Read the model definition and answer for the solid it produces. Units are mm, in the model's axes. Face numbers are marked on the shaded views. Coordinates: 2 decimals unless noted, no trailing zeros. Write each loop counter-clockwise with the first axis right and the second up, starting at its lowest first coordinate (ties: lowest second). Pieces come first, ordered by that corner, then holes. Notation, with made-up numbers: M 55.25,84.25 L 101.25,84.25 A19 cw 101.25,109.25 Z; hole C -15,6.5 d8. An arc over 180 degrees is marked long. Use a Markdown table: item, result. Add a question column.
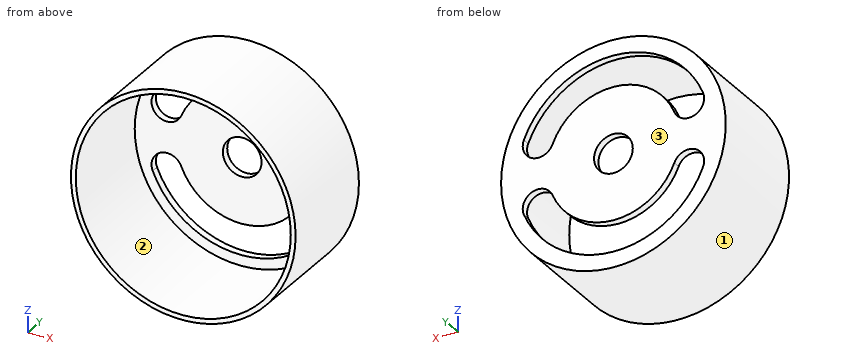
from build123d import *

# Parameters (mm, degrees)
F0_R     = 29
F1_DEPTH = 29
F2_R     = 27.75
F3_DEPTH = 27
F5_DEPTH = 2
F6_R     = 5
F7_DEPTH = 2


with BuildPart() as f1:
    # F0 (on Front) → F1 (new body)
    with BuildSketch(Plane.XZ):
        Circle(F0_R)
    extrude(amount=F1_DEPTH)

    # F2 (on face) → F3 (cut)
    with BuildSketch(Plane.XZ.offset(29)):
        Circle(F2_R)
    extrude(amount=-F3_DEPTH, mode=Mode.SUBTRACT)

    # F4 (on face) → F5 (cut)
    with BuildSketch(Plane(origin=(0, 0, 0), x_dir=(-1, 0, 0), z_dir=(0, 1, 0))):
        with BuildLine():
            ThreePointArc((-15.718109, -6.47619), (-20.940297, -4.301621), (-23.114866, -9.52381))
            ThreePointArc((-23.114866, -9.52381), (0, -25), (23.114866, -9.52381))
            ThreePointArc((23.114866, -9.52381), (20.940297, -4.301621), (15.718109, -6.47619))
            ThreePointArc((15.718109, -6.47619), (0, -17), (-15.718109, -6.47619))
        make_face()
        with BuildLine():
            ThreePointArc((23.114866, 9.52381), (0, 25), (-23.114866, 9.52381))
            ThreePointArc((-23.114866, 9.52381), (-20.940297, 4.301621), (-15.718109, 6.47619))
            ThreePointArc((-15.718109, 6.47619), (0, 17), (15.718109, 6.47619))
            ThreePointArc((15.718109, 6.47619), (20.940297, 4.301621), (23.114866, 9.52381))
        make_face()
    extrude(amount=-F5_DEPTH, mode=Mode.SUBTRACT)

    # F6 (on face) → F7 (cut)
    with BuildSketch(Plane(origin=(0, 0, 0), x_dir=(-1, 0, 0), z_dir=(0, 1, 0))):
        Circle(F6_R)
    extrude(amount=-F7_DEPTH, mode=Mode.SUBTRACT)


solid = f1.part
Item 1: Consider probe 1 along Z at (x, y) = (0, -0.8); probe 2 along Z at (x, y) = (0, -20.75); probe 3 along Z at (x, y) = (-24.5, -21.5). Determine where each line is inside the solid, lowest interval first.
Item 2: Find section D-D on x = -8. Give the vertices of the cut face in (y, z), then the cut area to 3 significant figures.
Item 3: Find section C-C on z = 8. Give the vertices of the cut face in (x, y).
Item 4: Determine the mould class of the marked faces 1, 2 and 3 for opening direction X: pulls with the +X half, pulls with the -X half, needs draft (parallel to the pull), parting line crosses it, or undercut.
Item 5: Find section A-A on z = 0. Give the vertices of the cut face in (x, y), then the cut area to 4 significant figures.
Item 6: Each of these flat-tipped pins is pushed along its axis until it touches: pin 1 (5 mm diameter, centred on x = -19, y = -22, fed in from +Z); pin 2 (12 mm diameter, centred on y = -12.5, z = 15, fed in from +X); pin 3 (4 mm diameter, centred on y = -22, z = -12.5, fed in from +X). Where does it stop, or does it pass through?
Item 7: Find section B-B on x = 0. Give the vertices of the cut face in (y, z), then the cut area to 4 significant figures.
Geometry says:
| question | item | result |
|---|---|---|
| 1 | probe 1 | z = -29 to -25, -17 to -5, 5 to 17, 25 to 29 |
| 1 | probe 2 | z = -29 to -27.75, 27.75 to 29 |
| 1 | probe 3 | z = -15.52 to -13.03, 13.03 to 15.52 |
| 2 | outline | M -29,-27.87 L 0,-27.87 L 0,-23.69 L -2,-23.69 L -2,-26.57 L -29,-26.57 Z; M -29,26.57 L -2,26.57 L -2,23.69 L 0,23.69 L 0,27.87 L -29,27.87 Z; M -2,-15 L 0,-15 L 0,15 L -2,15 Z |
| 2 | area | 147 mm2 |
| 3 | outline | M -27.87,-29 L -26.57,-29 L -26.57,-2 L -23.42,-2 L -23.42,0 L -27.87,0 Z; M -15,-2 L 15,-2 L 15,0 L -15,0 Z; M 23.42,-2 L 26.57,-2 L 26.57,-29 L 27.87,-29 L 27.87,0 L 23.42,0 Z |
| 4 | face 1 | parting line crosses it |
| 4 | face 2 | undercut |
| 4 | face 3 | needs draft |
| 5 | outline | M -29,-29 L -27.75,-29 L -27.75,-2 L -5,-2 L -5,0 L -29,0 Z; M 5,-2 L 27.75,-2 L 27.75,-29 L 29,-29 L 29,0 L 5,0 Z |
| 5 | area | 163.5 mm2 |
| 6 | pin 1 | stops at z = 23.85 |
| 6 | pin 2 | stops at x = 27.57 |
| 6 | pin 3 | stops at x = 27.03 |
| 7 | outline | M -29,-29 L 0,-29 L 0,-25 L -2,-25 L -2,-27.75 L -29,-27.75 Z; M -29,27.75 L -2,27.75 L -2,25 L 0,25 L 0,29 L -29,29 Z; M -2,-17 L 0,-17 L 0,-5 L -2,-5 Z; M -2,5 L 0,5 L 0,17 L -2,17 Z |
| 7 | area | 131.5 mm2 |
